The model under review builds one solid part; all positions refer to its coordinate system, in mm. A direction names the side the tool comes from. Coordinates: 2 decimals unless noted, no trailing zeros. Order: outer loops, then holes, each group sorted by start corner. A loop starts at its lowest first (then second) coordinate and runs counter-clockwise, first axis right, second up.
from build123d import *

# Parameters (mm, degrees)
SKETCH1_W           = 50.8
SKETCH1_H           = 25.4
SKETCH1_W_2         = 44.704
SKETCH1_H_2         = 19.304
BOSS_EXTRUDE1_DEPTH = 89.408
VARFILLET1_START    = -1
VARFILLET1_DEPTH    = 91
VARFILLET1_2_DEPTH  = 89.408


with BuildPart() as part:
    # Sketch1 → Boss-Extrude1 (new body)
    with BuildSketch(Plane.XY):
        with Locations((22.352, 9.652)):
            Rectangle(SKETCH1_W, SKETCH1_H)
        with Locations((22.352, 9.652)):
            Rectangle(SKETCH1_W_2, SKETCH1_H_2, mode=Mode.SUBTRACT)
    extrude(amount=BOSS_EXTRUDE1_DEPTH)

    # VarFillet1: read off the stored shape, not the designer's step
    # VarFillet1 outline → VarFillet1 (cut)
    with BuildSketch(Plane.XY.offset(VARFILLET1_START)):
        with BuildLine():
            Line((47.752, -3.048), (47.752, 0))
            add(Edge.make_bspline(
                [(47.752, 0), (47.752, -3.048), (44.704, -3.048)],
                knots=[0, 0, 0, 1, 1, 1], degree=2, weights=[1, 0.707106781, 1]))
            Line((44.704, -3.048), (47.752, -3.048))
        make_face()
        with BuildLine():
            add(Edge.make_bspline(
                [(44.704, 22.352), (47.752, 22.352), (47.752, 19.304)],
                knots=[0, 0, 0, 1, 1, 1], degree=2, weights=[1, 0.707106781, 1]))
            Line((47.752, 19.304), (47.752, 22.352))
            Line((47.752, 22.352), (44.704, 22.352))
        make_face()
        with BuildLine():
            Line((-3.048, -3.048), (0, -3.048))
            add(Edge.make_bspline(
                [(0, -3.048), (-3.048, -3.048), (-3.048, 0)],
                knots=[0, 0, 0, 1, 1, 1], degree=2, weights=[1, 0.707106781, 1]))
            Line((-3.048, 0), (-3.048, -3.048))
        make_face()
        with BuildLine():
            add(Edge.make_bspline(
                [(-3.048, 19.304), (-3.048, 22.352), (0, 22.352)],
                knots=[0, 0, 0, 1, 1, 1], degree=2, weights=[1, 0.707106781, 1]))
            Line((0, 22.352), (-3.048, 22.352))
            Line((-3.048, 22.352), (-3.048, 19.304))
        make_face()
    extrude(amount=VARFILLET1_DEPTH, mode=Mode.SUBTRACT)

    # VarFillet1 2 outline → VarFillet1 2 (add)
    with BuildSketch(Plane.XY):
        with BuildLine():
            add(Edge.make_bspline(
                [(3.048, 19.304), (0, 19.304), (0, 16.256)],
                knots=[0, 0, 0, 1, 1, 1], degree=2, weights=[1, 0.707106781, 1]))
            Line((3.048, 19.304), (0, 19.304))
            Line((0, 19.304), (0, 16.256))
        make_face()
        with BuildLine():
            Line((44.704, 19.304), (41.656, 19.304))
            add(Edge.make_bspline(
                [(44.704, 16.256), (44.704, 19.304), (41.656, 19.304)],
                knots=[0, 0, 0, 1, 1, 1], degree=2, weights=[1, 0.707106781, 1]))
            Line((44.704, 16.256), (44.704, 19.304))
        make_face()
        with BuildLine():
            add(Edge.make_bspline(
                [(0, 3.048), (0, 0), (3.048, 0)],
                knots=[0, 0, 0, 1, 1, 1], degree=2, weights=[1, 0.707106781, 1]))
            Line((0, 3.048), (0, 0))
            Line((0, 0), (3.048, 0))
        make_face()
        with BuildLine():
            Line((44.704, 0), (44.704, 3.048))
            add(Edge.make_bspline(
                [(41.656, 0), (44.704, 0), (44.704, 3.048)],
                knots=[0, 0, 0, 1, 1, 1], degree=2, weights=[1, 0.707106781, 1]))
            Line((41.656, 0), (44.704, 0))
        make_face()
    extrude(amount=VARFILLET1_2_DEPTH)


solid = part.part
(1) Wall thickness on line 1 (X direction, y = 14, z = 39); line 2 (Y direction, x = 10, z = 27); line 3 (Y direction, x = 2, z = 86): over which ranges is each line inside the solid? List them lowest first.
(2) Tool access review of faces 1 (the face through (22, 20, 89.408)), 2 (the face through (22, 19.304, 44)): name each direction out of +Z, -Z, +X, -X, +Y, -Y from which nothing blocks a thin tool from reaching the whole face with its end or side.
(3) Insertion check: pin 1 Ø8 at (x, y) = (13.5, 4.5) entering from +Z. The pin has a flat end and moves straight along its axis. Give the tip position at first contact, or say it passes through.
(4) Consider section B-B (y = 13.5). Give the boundary of the cut face in (x, z), then the cut area to 3 significant figures.
(5) The part is to be moulded in two halves that separate along Y. For faces 3 (the face through (0, 10, 44)), 4 (the face through (44.704, 10, 44)), 5 (the face through (-3.048, 10, 44)), 6 (the face through (22, -3.048, 44)), say which applies: +Y half, -Y half, draft (parallel to the pull), parting line (faces both ways), or undercut.
(6) Consider section A-A (x = 6.5). Give the boundary of the cut face in (y, z), then the cut area to 3 significant figures.
Findings:
1. line 1: x = -3.05 to 0, 44.7 to 47.75
1. line 2: y = -3.05 to 0, 19.3 to 22.35
1. line 3: y = -3.05 to 0.19, 19.12 to 22.35
2. face 1: +Z, +X, -X, +Y, -Y
2. face 2: +Z, -Z
3. pin 1: passes through
4. outline: (-3.05, 0) - (0, 0) - (0, 89.41) - (-3.05, 89.41) - close; (44.7, 0) - (47.75, 0) - (47.75, 89.41) - (44.7, 89.41) - close
4. area: 545 mm2
5. face 3: undercut
5. face 4: undercut
5. face 5: draft
5. face 6: -Y half
6. outline: (-3.05, 0) - (0, 0) - (0, 89.41) - (-3.05, 89.41) - close; (19.3, 0) - (22.35, 0) - (22.35, 89.41) - (19.3, 89.41) - close
6. area: 545 mm2
